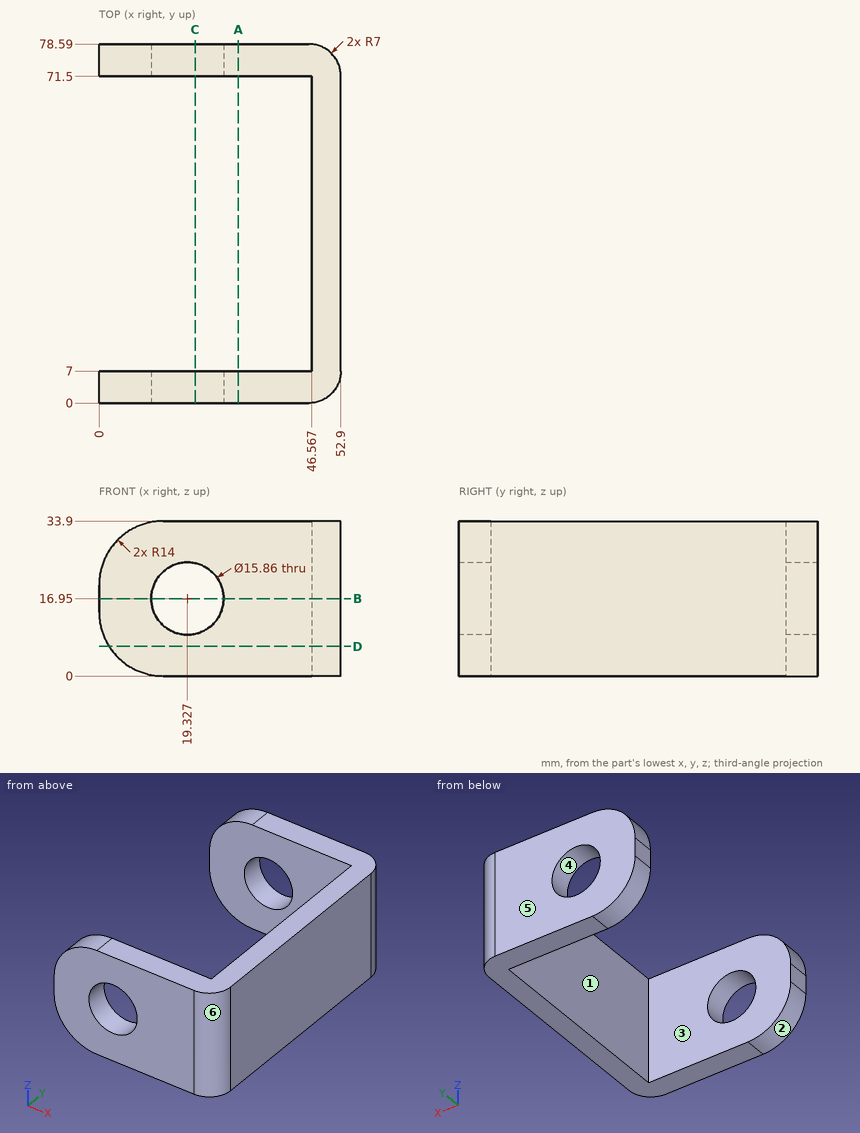
Can you work these out from the drawing? Everything is in mm from the part's minimum corner. A direction names the side the tool comes from. Coordinates: 2 decimals unless noted, no trailing zeros. Loops run counter-clockwise (first coordinate to the right, second up) from the corner with the lowest first, then second, coordinate; pieces in that order, holes last. Notation, with made-up numbers: M 37.25,78 L 43.25,78 A24 cw 43.25,101 Z; hole C 29.5,-30 d9. An arc over 180 degrees is marked long. Put each result on its own line as item: value. Start each with the question number.
(1) I need wall thicknesses on line 1 (Y direction, x = 43.5, z = 22.5); line 2 (X direction, y = 5, z = 16); line 3 (Y direction, x = 49, z = 2.5). Which ranges of each line are inside material? Lowest first, please. Write a range as from..to.
(2) Suppose I cut it at A-A on x = 30.5. Please give me the cut outline in (y, z), then the cut area to 3 significant figures.
(3) Thinking about a two-plate mould opening in Y: for the marked faces 3, 4, 5 and 6, which applies, pulls with the +Y half, pulls with the -Y half, needs draft (parallel to the pull), parting line crosses it, or undercut?
(4) Suppose I cut it at D-D on z = 6.5. Please give me the cut outline in (x, y).
(5) Suppose I cut it at C-C on x = 21. Please give me the cut outline in (y, z).
(6) Suppose I cut it at B-B on z = 16.95. Please give me the cut outline in (x, y), then the cut area to 3 significant figures.
(7) Will this pin go through, and if not, where does the flat tip stop? P1, Ø17, axis at y = 33, z = 10, coming from the -X side.
(8) For the marked faces 1 and 2, which set-ups out of +Z, -Z, +X, -X, +Y, -Y let a thin tool reach every point of the face, with its end or its side?
Solutions:
1. line 1: y = 0..7, 71.5..78.59
1. line 2: x = 0..11.45, 27.2..52.61
1. line 3: y = 0.72..77.87
2. outline: M 0,0 L 7,0 L 7,33.9 L 0,33.9 Z; M 71.5,0 L 78.59,0 L 78.59,33.9 L 71.5,33.9 Z
2. area: 478 mm2
3. face 3: undercut
3. face 4: needs draft
3. face 5: pulls with the +Y half
3. face 6: pulls with the -Y half
4. outline: M 2.18,0 L 45.9,0 A7 ccw 52.9,7 L 52.9,71.59 A7 ccw 45.9,78.59 L 2.18,78.59 L 2.18,71.5 L 46.57,71.5 L 46.57,7 L 2.18,7 Z
5. outline: M 0,0 L 7,0 L 7,9.2 L 0,9.2 Z; M 0,24.7 L 7,24.7 L 7,33.9 L 0,33.9 Z; M 71.5,0 L 78.59,0 L 78.59,9.2 L 71.5,9.2 Z; M 71.5,24.7 L 78.59,24.7 L 78.59,33.9 L 71.5,33.9 Z
6. outline: M 0,0 L 11.4,0 L 11.4,7 L 0,7 Z; M 0,71.5 L 11.4,71.5 L 11.4,78.59 L 0,78.59 Z; M 27.26,0 L 45.9,0 A7 ccw 52.9,7 L 52.9,71.59 A7 ccw 45.9,78.59 L 27.26,78.59 L 27.26,71.5 L 46.57,71.5 L 46.57,7 L 27.26,7 Z
6. area: 909 mm2
7. P1: stops at x = 46.57
8. face 1: +Z, -Z, -X
8. face 2: -Z, -X, +Y, -Y
